Design review of the part built by this model. Coordinates are the model's own, in mm. Face numbers are marked on the shaded views. Give positions to 0.01 mm unless a question says otherwise; leave off trailing zeros. Order: outer loops, then holes, each group sorted by start corner. A loop starts at its lowest first (then second) coordinate and runs counter-clockwise, first axis right, second up. Notation, with made-up numbers: (-15.75, 35) -> (32.25, 35) arc R23 ccw to (32.25, 48) -> close; hole circle Ø5 at (13.5, 70). An arc over 180 degrees is marked (long way). One line per item, written item: value. Start each with the question number.
1) Consider section C-C (y = 4). State the section outline as (x, z) points.
2) Consider section B-B (z = 0). State the section outline as (x, y) points, plus the area to 3 significant figures.
3) For pin 1 (1.5 mm diameter, centred on x = 1.5, y = 1.5, fed in from +Z), flat-tipped, find the tip position at first contact; note if it passes through.
4) The part is to be moulded in two halves that separate along Y. For the marked faces 1, 2, 3 and 4, say which applies: released by +Y, released by -Y, zero draft, split by the parting line, or undercut.
5) Consider section D-D (y = -2). State the section outline as (x, z) points.
6) Wall thickness on line 1 along X through (y, z) = (4.25, 0); line 2 along X through (y, z) = (1.5, -1.25); line 3 along Y through (x, z) = (1.75, 2.25): over which ranges is each line inside the solid? List them lowest first. Write a range as from..to.
7) Consider section A-A (y = 0.75). State the section outline as (x, z) points, plus the area to 3 significant figures.
from build123d import *

# Parameters (mm, degrees)
BOSS_EXTRUDE1_DEPTH = 8
SKETCH3_R           = 2.5
BOSS_EXTRUDE2_DEPTH = 1
SKETCH4_R           = 3
BOSS_EXTRUDE3_DEPTH = 4
FILLET1_R           = 0.5
SKETCH5_R           = 0.25
CUT_EXTRUDE1_DEPTH  = 100
CHAMFER1_SIZE       = 1
CHAMFER1_SIZE2      = 4.331475874
CHAMFER2_SIZE       = 0.25
CHAMFER2_SIZE2      = 0.333591751


with BuildPart() as part:
    # Sketch1 → Boss-Extrude1 (new body)
    with BuildSketch(Plane(origin=(0, 0, 0), x_dir=(1, 0, 0), z_dir=(0, 1, 0))):
        Polygon((-2.999284009, -1.725078384), (-0.0056803, -3.459995337), (2.993603709, -1.734916953), (2.999284009, 1.725078384), (0.0056803, 3.459995337), (-2.993603709, 1.734916953), align=None)
    extrude(amount=BOSS_EXTRUDE1_DEPTH)

    # Sketch2 → Cut-Revolve2 (revolve, cut)
    with BuildSketch(Plane.XY, mode=Mode.PRIVATE) as cut_revolve2_sk:
        Polygon((-0.4556803, 8), (-4.194310439, 2.85), (-4.194310439, 8), align=None)
    revolve(cut_revolve2_sk.sketch.rotate(Axis((-0.0056803, 8, 0), (0, -1, 0)), 90.188125981), axis=Axis((-0.0056803, 8, 0), (0, -1, 0)), mode=Mode.SUBTRACT)

    # Sketch3 → Boss-Extrude2 (add)
    with BuildSketch(Plane.XZ):
        with Locations(Location((0, 0, 0), (0, 0, 270))):
            Circle(SKETCH3_R)
    extrude(amount=BOSS_EXTRUDE2_DEPTH)

    # Sketch4 → Boss-Extrude3 (add)
    with BuildSketch(Plane.XZ.offset(1)):
        with Locations(Location((0, 0, 0), (0, 0, 270))):
            Circle(SKETCH4_R)
    extrude(amount=BOSS_EXTRUDE3_DEPTH)

    # Fillet1
    fillet1_edges = [part.edges().sort_by_distance(p)[0] for p in [
        (0, -5, 3),
    ]]
    fillet(fillet1_edges, radius=FILLET1_R)

    # Sketch5 → Cut-Extrude1 (cut)
    with BuildSketch(Plane(origin=(0, 8, 0), x_dir=(1, 0, 0), z_dir=(0, 1, 0))):
        with Locations(Location((0, 0, 0), (0, 0, 270))):
            Circle(SKETCH5_R)
    extrude(amount=-CUT_EXTRUDE1_DEPTH, mode=Mode.SUBTRACT)

    # Chamfer1
    chamfer1_edges = [part.edges().sort_by_distance(p)[0] for p in [
        (0, -5, -0.25),
    ]]
    chamfer1_side = [part.faces().sort_by_distance(p)[0] for p in [
        (0, -5, 2.429289322),
    ]]
    chamfer(chamfer1_edges, length=CHAMFER1_SIZE, length2=CHAMFER1_SIZE2, reference=chamfer1_side[0])

    # Chamfer2
    chamfer2_edges = [part.edges().sort_by_distance(p)[0] for p in [
        (0, -5, -1.25),
    ]]
    chamfer2_side = [part.faces().sort_by_distance(p)[0] for p in [
        (0, -2.834262063, -0.75),
    ]]
    chamfer(chamfer2_edges, length=CHAMFER2_SIZE, length2=CHAMFER2_SIZE2, reference=chamfer2_side[0])


solid = part.part
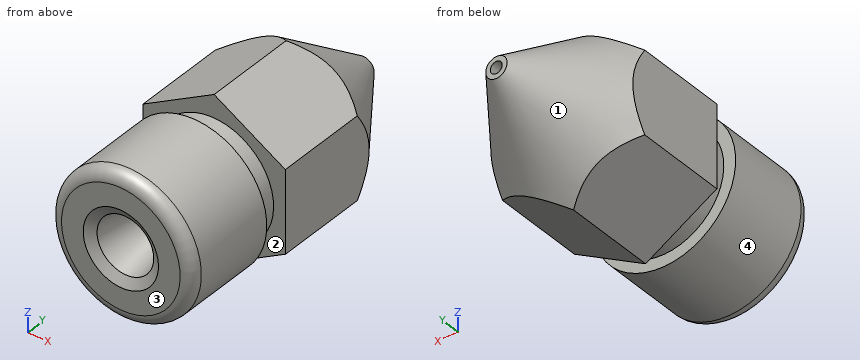
Checked values:
1. outline: (-3, 1.51) -> (-2.99, -1.52) arc R3.35 ccw to (-2.81, -1.84) -> (-0.19, -3.35) arc R3.35 ccw to (0.2, -3.35) -> (2.8, -1.84) arc R3.35 ccw to (3, -1.49) -> (2.99, 1.5) arc R3.35 ccw to (2.79, 1.85) -> (0.19, 3.35) arc R3.35 ccw to (-0.2, 3.35) -> (-2.81, 1.83) arc R3.35 ccw to start; hole circle Ø0.5 at (0, 0)
2. outline: (-3, -4.5) arc R0.5 ccw to (-2.5, -5) -> (-1.58, -5) -> (-1.19, -4.76) -> (-0.25, -0.67) -> (-0.25, 8) -> (-0.46, 8) -> (-3, 4.5) -> (-3, 0) -> (-2.5, 0) -> (-2.5, -1) -> (-3, -1) -> close; (0.25, -0.67) -> (1.19, -4.76) -> (1.58, -5) -> (2.5, -5) arc R0.5 ccw to (3, -4.5) -> (3, -1) -> (2.5, -1) -> (2.5, 0) -> (3, 0) -> (3, 4.48) -> (0.44, 8) -> (0.25, 8) -> close
2. area: 57.0 mm^2
3. pin 1: stops at z = 3.03
4. face 1: released by +Y
4. face 2: undercut
4. face 3: released by -Y
4. face 4: zero draft
5. outline: circle Ø6 at (0, 0); hole circle Ø1.11 at (0, 0)
6. line 1: x = -3..-0.25, 0.25..3
6. line 2: x = -2.99..3
6. line 3: y = -4.86..-1, 0..4.69
7. outline: (-3, 1.73) -> (-2.99, -1.73) -> (0.01, -3.46) -> (3, -1.73) -> (2.99, 1.73) -> (-0.01, 3.46) -> close; hole circle Ø0.5 at (0, 0)
7. area: 30.9 mm^2
